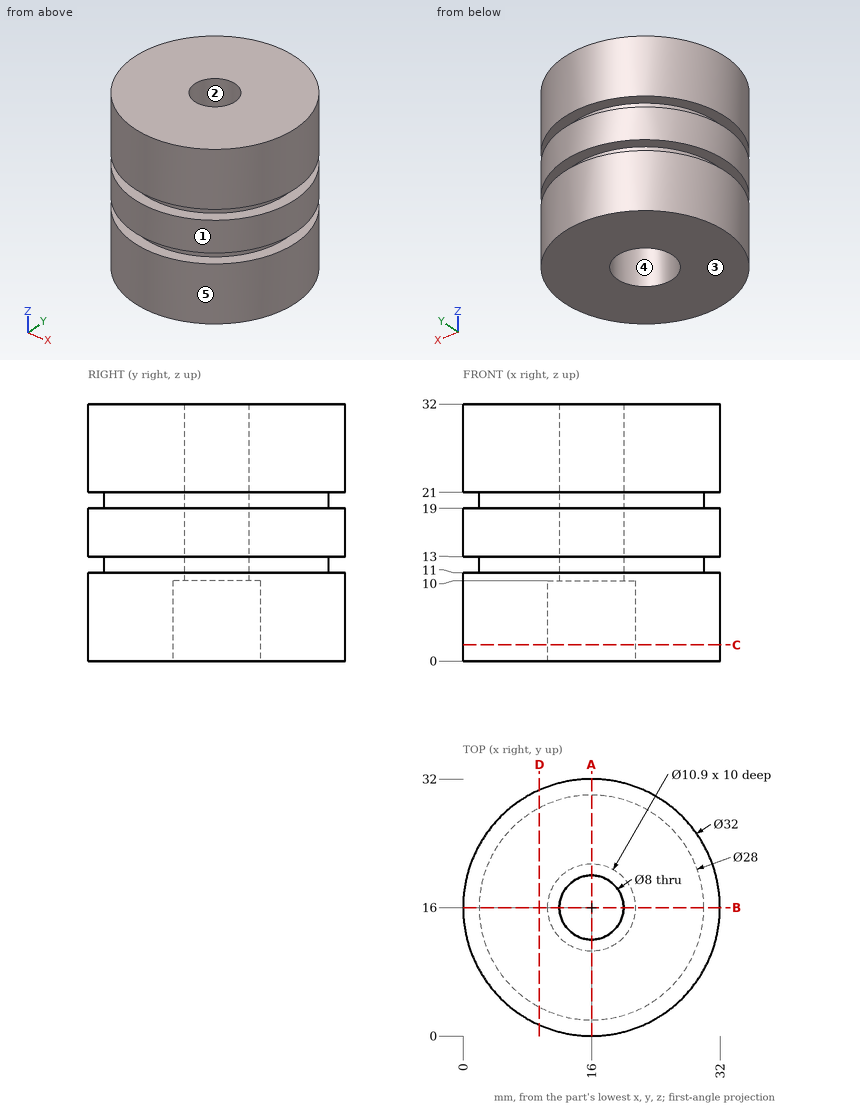
Geometry: see drawing. Coordinates: mm, zero at the bounding-box minimum. A direction names the side the tool comes from. Coordinates: 2 decimals unless noted, no trailing zeros. Order: outer loops, then holes, each group sorted by start corner. A loop starts at its lowest first (then second) coordinate and runs counter-clockwise, first axis right, second up. Notation, with made-up numbers: (-2.5, 13) - (30.5, 13) arc R3 ccw to (30.5, 17) - close; hole circle Ø3 at (67, 82). An arc over 180 degrees is marked (long way). Use one line per item in the form item = value.
1) Set-up query: the marked faces 4 and 5. Return all of +Z, -Z, +X, -X, +Y, -Y with unobstructed straight access to the full face (end or side cutting, diameter ignored); none if empty.
Solutions:
face_4 = -Z
face_5 = +Z, -Z
2) Pin query (flat end, axial travel): pin 1 (8 mm diameter, centred on x = 22, z = 23.5, fed in from -Y); pin 2 (17.5 mm diameter, centred on x = 16, y = 16, fed in from +Z); pin 3 (3 mm diameter, centred on y = 19, z = 12.5, fed in from -X); pin 4 (5 mm diameter, centred on x = 6.5, z = 22.5, fed in from -Y). Return the tip coordinate at first contact, or that it passes through.
Solutions:
pin_1 = 0.13
pin_2 = 32
pin_3 = 0.08
pin_4 = 1.61
3) Section D-D (x = 9.5). Return loops of the section in (y, z).
Solutions:
outline = (1.38, 0) - (30.62, 0) - (30.62, 11) - (28.4, 11) - (28.4, 13) - (30.62, 13) - (30.62, 19) - (28.4, 19) - (28.4, 21) - (30.62, 21) - (30.62, 32) - (1.38, 32) - (1.38, 21) - (3.6, 21) - (3.6, 19) - (1.38, 19) - (1.38, 13) - (3.6, 13) - (3.6, 11) - (1.38, 11) - close
4) Ray query, L1, parallel to Y at x = 16, z = 20.5; L2, parallel to Z at x = 28, y = 24; L3, parallel to Y at x = 16, z = 15. Return the intervals inside material, ascending.
Solutions:
L1 = 2 to 12, 20 to 30
L2 = 0 to 11, 13 to 19, 21 to 32
L3 = 0 to 12, 20 to 32
5) Mould query, pull axis Y, two halves, no side actions, for the marked faces 1, 2 and 3. Classes: +Y half, -Y half, draft (parallel to the pull), parting line (faces both ways), or undercut.
Solutions:
face_1 = parting line
face_2 = undercut
face_3 = draft
6) Section C-C (z = 2). Return loops of the section in (x, y), then the cut area to 3 significant figures.
Solutions:
outline = circle Ø32 at (16, 16); hole circle Ø10.9 at (16, 16)
area = 711 mm^2
7) Section A-A (x = 16). Return loops of the section in (y, z), then the cut area to 3 significant figures.
Solutions:
outline = (0, 0) - (10.55, 0) - (10.55, 10) - (12, 10) - (12, 32) - (0, 32) - (0, 21) - (2, 21) - (2, 19) - (0, 19) - (0, 13) - (2, 13) - (2, 11) - (0, 11) - close; (20, 10) - (21.45, 10) - (21.45, 0) - (32, 0) - (32, 11) - (30, 11) - (30, 13) - (32, 13) - (32, 19) - (30, 19) - (30, 21) - (32, 21) - (32, 32) - (20, 32) - close
area = 723 mm^2
